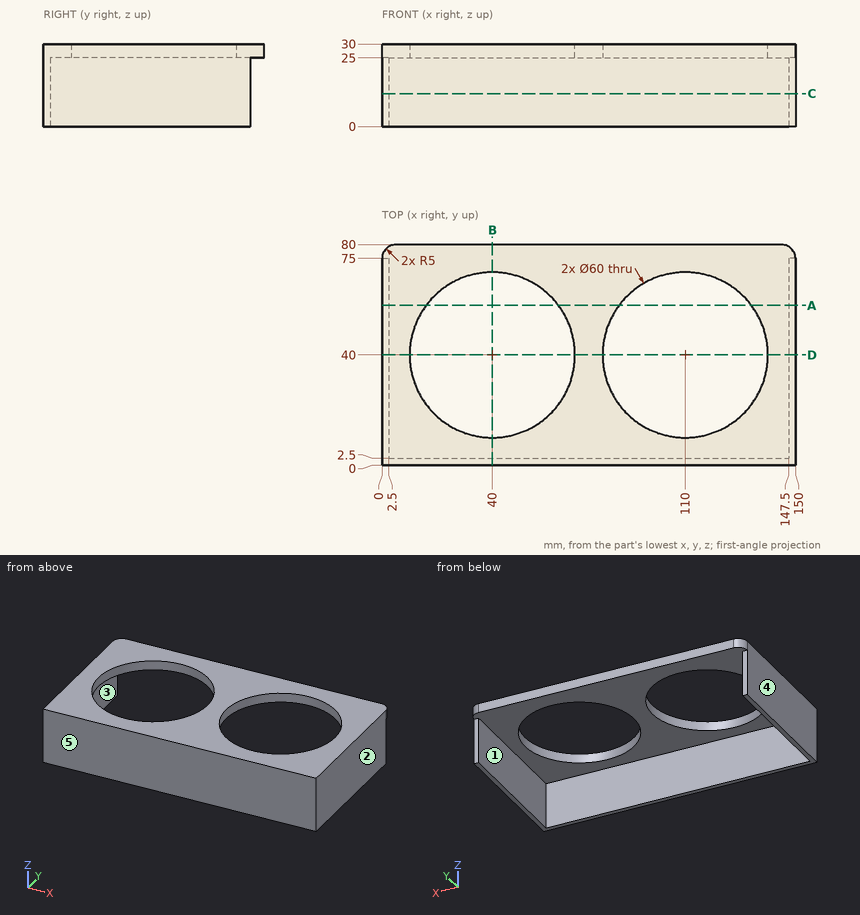
Study the drawing (mm; zero at the part's minimum x, y, z) and answer. A direction names the side the tool comes from. Give positions to 0.01 mm unless a question says otherwise; leave off trailing zeros. Loops run counter-clockwise (first coordinate to the right, second up) from the corner with the lowest first, then second, coordinate; pieces in that order, holes last. Notation, with made-up numbers: (-36.5, 75) - (-5.5, 75) arc R17 cw to (-5.5, 79) - close; hole circle Ø3 at (10, 58.5). An arc over 180 degrees is marked (long way). Answer in a Markdown table with one row per item. Add a question column.
Q1. The part is cut by section A-A (y = 58). Determine the outline of the cut face in (x, z), and give its area (3 significant figures).
Q2. Consider line 1 along Y through (x, z) = (110, 27.35); line 2 along X through (y, z) = (39, 10); line 3 along Z through (x, y) = (140, 21.5). Determine where each line is inside the solid, lowest interval first.
Q3. The part is cut by section D-D (y = 40). Determine the outline of the cut face in (x, z).
Q4. The part is cut by section B-B (x = 40). Determine the outline of the cut face in (y, z), and give its area (4 significant figures).
Q5. The part is cut by section C-C (z = 12). Determine the outline of the cut face in (x, y).
Q6. A tool of negligible diameter and unlimited length cuts with its end or side. For the marked faces 1 and 2, from which of +Z, -Z, +X, -X, +Y, -Y can it reach the whole face along a straight path? Write none if from no direction.
Q7. This flat-tipped pin is pushed along its axis until it touches: P1, Ø0.8, axis at x = 1, z = 11.5, coming from the +Y side. Where does it stop, or does it pass through?
Q8. Determine the mould class of the marked faces 3, 4 and 5 for opening direction X: released by +X, released by -X, zero draft, split by the parting line, or undercut.
Solution:
| question | item | result |
|---|---|---|
| 1 | outline | (0, 0) - (2.5, 0) - (2.5, 25) - (16, 25) - (16, 30) - (0, 30) - close; (64, 25) - (86, 25) - (86, 30) - (64, 30) - close; (134, 25) - (147.5, 25) - (147.5, 0) - (150, 0) - (150, 30) - (134, 30) - close |
| 1 | area | 395 mm² |
| 2 | line 1 | y = 0 to 10, 70 to 80 |
| 2 | line 2 | x = 0 to 2.5, 147.5 to 150 |
| 2 | line 3 | z = 25 to 30 |
| 3 | outline | (0, 0) - (2.5, 0) - (2.5, 25) - (10, 25) - (10, 30) - (0, 30) - close; (70, 25) - (80, 25) - (80, 30) - (70, 30) - close; (140, 25) - (147.5, 25) - (147.5, 0) - (150, 0) - (150, 30) - (140, 30) - close |
| 4 | outline | (0, 0) - (2.5, 0) - (2.5, 25) - (10, 25) - (10, 30) - (0, 30) - close; (70, 25) - (80, 25) - (80, 30) - (70, 30) - close |
| 4 | area | 162.5 mm² |
| 5 | outline | (0, 0) - (150, 0) - (150, 75) - (147.5, 75) - (147.5, 2.5) - (2.5, 2.5) - (2.5, 75) - (0, 75) - close |
| 6 | face 1 | -Z, +Y |
| 6 | face 2 | +Z, -Z, +X, +Y, -Y |
| 7 | P1 | stops at y = 75 |
| 8 | face 3 | undercut |
| 8 | face 4 | released by -X |
| 8 | face 5 | zero draft |
